Check sheet for the modelled part. Datum: model origin and axes. Units: mm. Face numbers are marked on the shaded views. A direction names the side the tool comes from. Round coordinates to 2 decimals unless told otherwise and drop trailing zeros. Order: outer loops, then holes, each group sorted by start corner. A loop starts at its lowest first (then second) coordinate and runs counter-clockwise, first axis right, second up. Notation, with made-up numbers: (-39.5, 40) -> (-29.5, 40) arc R15 ccw to (-29.5, 46) -> close; hole circle Ø11 at (17, -1.75). An arc over 180 degrees is marked (long way). Answer in a Markdown table with one row per item.
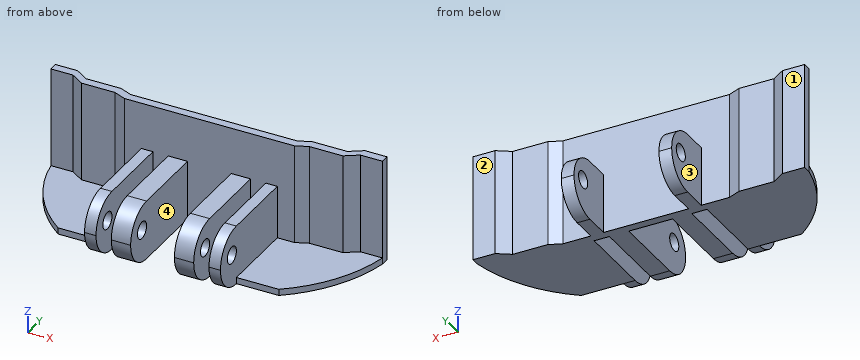
```python
from build123d import *

# Parameters (mm, degrees)
SKETCH2_W                 = 5
SKETCH2_H                 = 25
BOSS_EXTRUDE1_DEPTH       = 14
BOSS_EXTRUDE1_2_DEPTH     = 14
BOSS_EXTRUDE3_DEPTH       = 25
SKETCH5_W                 = 3
SKETCH5_H                 = 13
BOSS_EXTRUDE4_DEPTH       = 14
SKETCH7_W                 = 3
SKETCH7_H                 = 25
BOSS_EXTRUDE5_DEPTH       = 14
SKETCH15_W                = 0.3
SKETCH15_H                = 14
CUT_EXTRUDE2_DEPTH        = 25
SKETCH16_W                = 0.15
SKETCH16_H                = 14
CUT_EXTRUDE3_DEPTH        = 25
FILLET1_R                 = 7
F_4_0MM_DOWEL_HOLE2_D     = 4
FILLET2_R                 = 7
F_4_0MM_DOWEL_HOLE1_D     = 4
F_4_0MM_DOWEL_HOLE1_DEPTH = 26
F_4_0MM_DOWEL_HOLE1_TIP   = 1.201721238
BOSS_EXTRUDE6_DEPTH       = 1.5


with BuildPart() as part:
    # Sketch2 → Boss-Extrude1 (new body)
    with BuildSketch(Plane.XY):
        with Locations((-7.5, -6.5)):
            Rectangle(SKETCH2_W, SKETCH2_H)
    extrude(amount=BOSS_EXTRUDE1_DEPTH)



with BuildPart() as body_2:
    # Sketch2 → Boss-Extrude1 2 (new body)
    with BuildSketch(Plane.XY):
        with Locations((7.5, -6.5)):
            Rectangle(SKETCH2_W, SKETCH2_H)
    extrude(amount=BOSS_EXTRUDE1_2_DEPTH)


with BuildPart() as part_1:
    add(part.part)

    add(body_2.part)  # Boss-Extrude3 merges body 2
    # Sketch4 → Boss-Extrude3 (add)
    with BuildSketch(Plane.XY):
        Polygon((-26, 9.206366686), (-30.765993712, 9.206366686), (-33.831204342, 11.206366686), (-39.037863495, 11.206366686), (-39.037863495, 9.206366686), (-33.831204342, 9.206366686), (-30.765993712, 7.206366686), (-26, 7.206366686), align=None)
        Polygon((22.901603942, 7.206366686), (26, 7.206366686), (26, 9.206366686), (22.502408858, 9.206366686), (19.600804916, 8), (10, 8), (-10, 8), (-19.600804916, 8), (-22.502408858, 9.206366686), (-26, 9.206366686), (-26, 7.206366686), (-22.901603942, 7.206366686), (-20, 6), (-10, 6), (10, 6), (20, 6), align=None)
        Polygon((26, 7.206366686), (26, 9.206366686), (30.765993712, 9.206366686), (33.831204342, 11.206366686), (39.037863495, 11.206366686), (39.037863495, 9.206366686), (33.831204342, 9.206366686), (30.765993712, 7.206366686), align=None)
    extrude(amount=BOSS_EXTRUDE3_DEPTH)

    # Sketch5 → Boss-Extrude4 (add)
    with BuildSketch(Plane.XY):
        with Locations((-11.5, 14.5)):
            Rectangle(SKETCH5_W, SKETCH5_H)
        with Locations((11.5, 14.5)):
            Rectangle(SKETCH5_W, SKETCH5_H)
    extrude(amount=BOSS_EXTRUDE4_DEPTH)

    # Sketch7 → Boss-Extrude5 (add)
    with BuildSketch(Plane.XY):
        with Locations((-14.5, -6.5)):
            Rectangle(SKETCH7_W, SKETCH7_H)
        with Locations((14.5, -6.5)):
            Rectangle(SKETCH7_W, SKETCH7_H)
    extrude(amount=BOSS_EXTRUDE5_DEPTH)

    # Sketch15 → Cut-Extrude2 (cut)
    with BuildSketch(Plane.XZ.offset(19)):
        with Locations((-9.85, 7)):
            Rectangle(SKETCH15_W, SKETCH15_H)
        with Locations((9.85, 7)):
            Rectangle(SKETCH15_W, SKETCH15_H)
        with Locations((-13.15, 7)):
            Rectangle(SKETCH15_W, SKETCH15_H)
        with Locations((13.15, 7)):
            Rectangle(SKETCH15_W, SKETCH15_H)
    extrude(amount=-CUT_EXTRUDE2_DEPTH, mode=Mode.SUBTRACT)

    # Sketch16 → Cut-Extrude3 (cut)
    with BuildSketch(Plane.XZ.offset(19)):
        with Locations((-5.075, 7)):
            Rectangle(SKETCH16_W, SKETCH16_H)
        with Locations((5.075, 7)):
            Rectangle(SKETCH16_W, SKETCH16_H)
    extrude(amount=-CUT_EXTRUDE3_DEPTH, mode=Mode.SUBTRACT)

    # Fillet1
    fillet1_edges = [part_1.edges().sort_by_distance(p)[0] for p in [
        (7.425, -19, 0),
        (7.425, -19, 14),
        (-7.425, -19, 0),
        (-7.425, -19, 14),
        (-14.65, -19, 0),
        (-14.65, -19, 14),
        (14.65, -19, 14),
        (14.65, -19, 0),
    ]]
    fillet(fillet1_edges, radius=FILLET1_R - 0.0001)  # a hair under: the kernel refuses the full size

    # Ø4.0mm Dowel Hole2 (through all)
    with Locations(Plane(origin=(16, 0, 0), x_dir=(0, 0, -1), z_dir=(1, 0, 0))):
        with Locations((-8, -14)):
            Hole(F_4_0MM_DOWEL_HOLE2_D / 2)

    # Fillet2
    fillet2_edges = [part_1.edges().sort_by_distance(p)[0] for p in [
        (-11.5, 21, 0),
        (-11.5, 21, 14),
        (11.5, 21, 0),
        (11.5, 21, 14),
    ]]
    fillet(fillet2_edges, radius=FILLET2_R - 0.0001)  # a hair under: the kernel refuses the full size

    # Ø4.0mm Dowel Hole1
    with Locations(Plane(origin=(13, 0, 0), x_dir=(0, 0, -1), z_dir=(1, 0, 0))):
        with Locations((-8, 17)):
            Hole(F_4_0MM_DOWEL_HOLE1_D / 2, depth=F_4_0MM_DOWEL_HOLE1_DEPTH)
            with Locations((0, 0, -(F_4_0MM_DOWEL_HOLE1_DEPTH + F_4_0MM_DOWEL_HOLE1_TIP / 2))):  # 118° drill point
                Cone(0, F_4_0MM_DOWEL_HOLE1_D / 2, F_4_0MM_DOWEL_HOLE1_TIP, mode=Mode.SUBTRACT)

    # Sketch14 → Boss-Extrude6 (add)
    with BuildSketch(Plane.XY):
        with BuildLine():
            Line((-22.901603942, 7.206366686), (-30.765993712, 7.206366686))
            Line((-30.765993712, 7.206366686), (-33.831204342, 9.206366686))
            Line((-33.831204342, 9.206366686), (-39.037863495, 9.206366686))
            ThreePointArc((-39.037863495, 9.206366686), (-34.518223809, -2.625999259), (-26, -12))
            Line((-26, -12), (-16, -12))
            Line((-16, -12), (-16, 6))
            Line((-16, 6), (-20, 6))
            Line((-20, 6), (-22.901603942, 7.206366686))
        make_face()
        with BuildLine():
            Line((20, 6), (16, 6))
            Line((16, 6), (16, -12))
            Line((16, -12), (26, -12))
            ThreePointArc((26, -12), (34.518223809, -2.625999259), (39.037863495, 9.206366686))
            Line((39.037863495, 9.206366686), (33.831204342, 9.206366686))
            Line((33.831204342, 9.206366686), (30.765993712, 7.206366686))
            Line((30.765993712, 7.206366686), (22.901603942, 7.206366686))
            Line((22.901603942, 7.206366686), (20, 6))
        make_face()
    extrude(amount=BOSS_EXTRUDE6_DEPTH)


solid = part_1.part
```
(1) Section check C-C on x = -18.5. Record the boundary of the cut face in (y, z), plus the area to 3 significant figures.
Solutions:
| item | result |
|---|---|
| outline | (-12, 0) -> (8, 0) -> (8, 25) -> (6, 25) -> (6, 1.5) -> (-12, 1.5) -> close |
| area | 77.0 mm^2 |
(2) Tool access check on the marked faces 1, 2, 3 and 4. Record the directions out of +Z, -Z, +X, -X, +Y, -Y that give a thin tool (end or side, any length) a straight path to the whole face; none if there is none.
Solutions:
| item | result |
|---|---|
| face 1 | +Z, -Z, -X, +Y |
| face 2 | +Z, -Z, +X, +Y |
| face 3 | +Z, -Z, +Y |
| face 4 | +Z, -Z, -Y |
(3) Section check D-D on z = 8. Give the number of separate pieces and of enclosed holes in the cut face, plus the area to 3 significant figures.
Solutions:
| item | result |
|---|---|
| separate pieces | 7 |
| enclosed holes | 0 |
| area | 514 mm^2 |
(4) Section check A-A on y = 16. Record the boundary of the cut face in (x, z).
Solutions:
| item | result |
|---|---|
| outline | (-13, 0.29) -> (-10, 0.29) -> (-10, 6.27) -> (-13, 6.27) -> close; (-13, 9.73) -> (-10, 9.73) -> (-10, 13.71) -> (-13, 13.71) -> close; (10, 0.29) -> (13, 0.29) -> (13, 6.27) -> (10, 6.27) -> close; (10, 9.73) -> (13, 9.73) -> (13, 13.71) -> (10, 13.71) -> close |
(5) Depth check by flat-ended pin: pin 1 Ø7 at (y, z) = (-9.5, 7) entering from +X; pin 2 Ø10 at (x, z) = (-27, 9.5) entering from -Y; pin 3 Ø2.5 at (x, y) = (8, -3) entering from +Z. Enter the tip coordinate at first touch or a pass-through.
Solutions:
| item | result |
|---|---|
| pin 1 | x = 16 |
| pin 2 | y = 6.83 |
| pin 3 | z = 14 |
(6) Scan lines: probe 1 along X at (y, z) = (-4, 13.75); probe 2 along X at (y, z) = (15, 13); probe 3 along X at (y, z) = (9, 11). Record each from-to range of solid material in increasing order. Write a range as from..to.
Solutions:
| item | result |
|---|---|
| probe 1 | -16..-13.3, -9.7..-5.15, 5.15..9.7, 13.3..16 |
| probe 2 | -13..-10, 10..13 |
| probe 3 | -33.51..-22.01, -13..-10, 10..13, 22.01..33.51 |
(7) Section check B-B on z = 18.5. Record the boundary of the cut face in (x, y), plus the area to 3 significant figures.
Solutions:
| item | result |
|---|---|
| outline | (-39.04, 9.21) -> (-33.83, 9.21) -> (-30.77, 7.21) -> (-22.9, 7.21) -> (-20, 6) -> (20, 6) -> (22.9, 7.21) -> (30.77, 7.21) -> (33.83, 9.21) -> (39.04, 9.21) -> (39.04, 11.21) -> (33.83, 11.21) -> (30.77, 9.21) -> (22.5, 9.21) -> (19.6, 8) -> (-19.6, 8) -> (-22.5, 9.21) -> (-30.77, 9.21) -> (-33.83, 11.21) -> (-39.04, 11.21) -> close |
| area | 157 mm^2 |
